```python
from build123d import *
from OCP.BRepFilletAPI import BRepFilletAPI_MakeChamfer

# Parameters (mm, degrees)
ESBO_O1_W                = 0.64
ESBO_O1_H                = 11.6
RESSALTO_EXTRUS_O1_DEPTH = 0.32
ESBO_O2_W                = 2.54
ESBO_O2_H                = 2.54
RESSALTO_EXTRUS_O2_DEPTH = 1.27
CHANFRO1_SIZE            = 0.15
CHANFRO1_SIZE2           = 0.26
CHANFRO2_SIZE            = 0.26
CHANFRO2_SIZE2           = 0.15
CHANFRO3_SIZE            = 0.25


with BuildPart() as part:
    # Esboço1 → Ressalto-extrusão1 (new, symmetric)
    with BuildSketch(Plane.XY):
        Rectangle(ESBO_O1_W, ESBO_O1_H)
    extrude(amount=RESSALTO_EXTRUS_O1_DEPTH, both=True)

    # Esboço2 → Ressalto-extrusão2 (add, symmetric)
    with BuildSketch(Plane.XY):
        with Locations((0, 1.47)):
            Rectangle(ESBO_O2_W, ESBO_O2_H)
    extrude(amount=RESSALTO_EXTRUS_O2_DEPTH, both=True)

    # Chanfro1
    chanfro1_edges = [part.edges().sort_by_distance(p)[0] for p in [
        (0, 5.8, -0.32),
        (-0.32, 5.8, 0),
        (0.32, 5.8, 0),
        (0, 5.8, 0.32),
    ]]
    chanfro1_side = [part.faces().sort_by_distance(p)[0] for p in [
        (0, 5.8, 0),
    ]]
    chamfer(chanfro1_edges, length=CHANFRO1_SIZE, length2=CHANFRO1_SIZE2, reference=chanfro1_side[0])

    # Chanfro2: one chamfer whose edges measure the first distance from different faces: ONE call of the kernel's chamfer builder (chamfer() names one face for all edges)
    chanfro2_edges_1 = [part.edges().sort_by_distance(p)[0] for p in [
        (0, -5.8, 0.32),
    ]]
    chanfro2_side_1 = [part.faces().sort_by_distance(p)[0] for p in [
        (0, -2.8, 0.32),
    ]]
    chanfro2_edges_2 = [part.edges().sort_by_distance(p)[0] for p in [
        (0, -5.8, -0.32),
    ]]
    chanfro2_side_2 = [part.faces().sort_by_distance(p)[0] for p in [
        (0, -2.8, -0.32),
    ]]
    chanfro2_edges_3 = [part.edges().sort_by_distance(p)[0] for p in [
        (0.32, -5.8, 0),
    ]]
    chanfro2_side_3 = [part.faces().sort_by_distance(p)[0] for p in [
        (0.32, -2.8, 0),
    ]]
    chanfro2_edges_4 = [part.edges().sort_by_distance(p)[0] for p in [
        (-0.32, -5.8, 0),
    ]]
    chanfro2_side_4 = [part.faces().sort_by_distance(p)[0] for p in [
        (-0.32, -2.8, 0),
    ]]
    chanfro2 = BRepFilletAPI_MakeChamfer(part.part.solid().wrapped)
    for e in chanfro2_edges_1:
        chanfro2.Add(CHANFRO2_SIZE, CHANFRO2_SIZE2, e.wrapped, chanfro2_side_1[0].wrapped)  # the first distance lies on this face
    for e in chanfro2_edges_2:
        chanfro2.Add(CHANFRO2_SIZE, CHANFRO2_SIZE2, e.wrapped, chanfro2_side_2[0].wrapped)  # the first distance lies on this face
    for e in chanfro2_edges_3:
        chanfro2.Add(CHANFRO2_SIZE, CHANFRO2_SIZE2, e.wrapped, chanfro2_side_3[0].wrapped)  # the first distance lies on this face
    for e in chanfro2_edges_4:
        chanfro2.Add(CHANFRO2_SIZE, CHANFRO2_SIZE2, e.wrapped, chanfro2_side_4[0].wrapped)  # the first distance lies on this face
    add(Compound.cast(chanfro2.Shape()), mode=Mode.REPLACE)

    # Chanfro3
    chanfro3_edges = [part.edges().sort_by_distance(p)[0] for p in [
        (-1.27, 1.47, -1.27),
        (-1.27, 2.74, 0),
        (0, 0.2, -1.27),
        (-1.27, 0.2, 0),
        (1.27, 1.47, -1.27),
        (1.27, 0.2, 0),
        (0, 2.74, -1.27),
        (1.27, 2.74, 0),
        (-1.27, 1.47, 1.27),
        (0, 0.2, 1.27),
        (1.27, 1.47, 1.27),
        (0, 2.74, 1.27),
    ]]
    chamfer(chanfro3_edges, length=CHANFRO3_SIZE)


solid = part.part
```
Model file for the job. Use its own axes, mm. Coordinates: 2 decimals unless noted, no trailing zeros. Loops run counter-clockwise (first coordinate to the right, second up) from the corner with the lowest first, then second, coordinate; pieces in that order, holes last. Notation, with made-up numbers: (-28.5, 87.25) -> (0.5, 87.25) arc R36 cw to (0.5, 123.25) -> close; hole circle Ø5 at (-10, 42). An arc over 180 degrees is marked (long way). Answer as a JSON object with one key per item and string values.
Q1. Cut at B-B (x = -0.55). List the corners of the cut face in (y, z).
Report:
{"outline": "(0.2, -1.02) -> (0.45, -1.27) -> (2.49, -1.27) -> (2.74, -1.02) -> (2.74, 1.02) -> (2.49, 1.27) -> (0.45, 1.27) -> (0.2, 1.02) -> close"}
Q2. Cut at C-C (y = 3.25). List the corners of the cut face in (x, z), and give its area (3 significant figures).
Report:
{"outline": "(-0.32, -0.32) -> (0.32, -0.32) -> (0.32, 0.32) -> (-0.32, 0.32) -> close", "area": "0.410 mm2"}
Q3. Pull direction Y, two halves, no side cores. Call faces 1 (the flat face through (0, 0.2, 0.5)), 2 (the flat face through (0, 1, 1.27)), 3 (the flat face through (0, 2.74, 0.5)): released by +Y, released by -Y, zero draft, split by the parting line, or undercut.
Report:
{"face 1": "released by -Y", "face 2": "zero draft", "face 3": "released by +Y"}
Q4. Cut at A-A (y = 2). List the corners of the cut face in (x, z), and give its area (3 significant figures).
Report:
{"outline": "(-1.27, -1.02) -> (-1.02, -1.27) -> (1.02, -1.27) -> (1.27, -1.02) -> (1.27, 1.02) -> (1.02, 1.27) -> (-1.02, 1.27) -> (-1.27, 1.02) -> close", "area": "6.33 mm2"}
Q5. Probe probe 1 along Y at (x, z) = (-0.65, -1); probe 2 along Z at (x, y) = (0.15, -3.5). List the from-to ranges inside material, lowest first.
Report:
{"probe 1": "y = 0.2 to 2.74", "probe 2": "z = -0.32 to 0.32"}
Q6. Flat gauge pins, fed straight in: P1, Ø0.7, axis at x = 0, y = 4, coming from the +Z side; P2, Ø0.6, axis at x = 0, z = -0.5, coming from the -Y side; P3, Ø0.5, axis at y = 4.5, z = 0, coming from the -X side. Where does each tip first touch, or does it go through?
Report:
{"P1": "stops at z = 0.32", "P2": "stops at y = -5.75", "P3": "stops at x = -0.32"}
